```python
from build123d import *


with BuildPart() as f3:
    # F3: sweep along a path in F0
    with BuildLine(Plane.XZ) as f3_path:
        Line((-75.8256912231, 30), (74.0892291069, 30))
        ThreePointArc((74.0892291069, 30), (104.0892291069, 0), (74.0892291069, -30))
        Line((74.0892291069, -30), (-75.8256912231, -30))
        ThreePointArc((-75.8256912231, -30), (-105.8256912231, 0), (-75.8256912231, 30))
    # F2 (on plane+point) → F3 (sweep)
    with BuildSketch(Plane.YZ.offset(74.0892291069)):
        Polygon((1.443375673, 35), (2.8867513459, 32.5), (4.3301270189, 35), align=None)
        Polygon((-1.443375673, 35), (1.443375673, 35), (0, 37.5), align=None)
        Polygon((-4.3301270189, 35), (-2.8867513459, 32.5), (-1.443375673, 35), align=None)
        Polygon((-4.3301270189, 30), (-1.443375673, 30), (-2.8867513459, 32.5), align=None)
        Polygon((0, 27.5), (1.443375673, 30), (-1.443375673, 30), align=None)
        Polygon((1.443375673, 30), (4.3301270189, 30), (2.8867513459, 32.5), align=None)
        Polygon((-1.443375673, 30), (1.443375673, 30), (2.8867513459, 32.5), (1.443375673, 35), (-1.443375673, 35), (-2.8867513459, 32.5), align=None)
    sweep(path=f3_path.line)


solid = f3.part
```
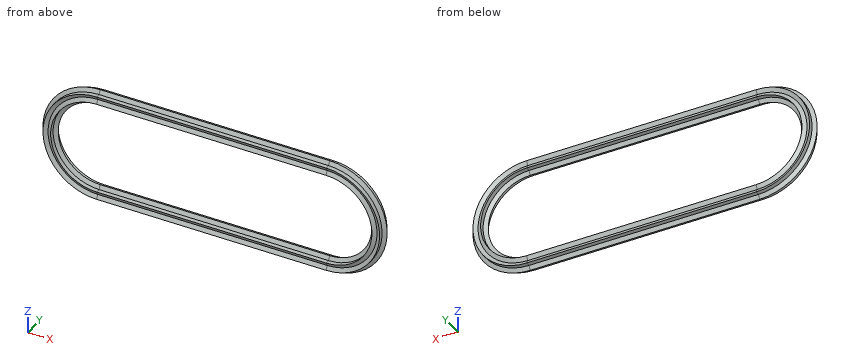
The listing builds one solid part. Answer for the finished solid, in the listing's coordinates (mm). Round coordinates to 2 decimals unless told otherwise and drop trailing zeros. Write each loop counter-clockwise with the first axis right and the second up, starting at its lowest first coordinate (ties: lowest second). Pieces come first, ordered by that corner, then holes. Notation, with made-up numbers: (22, 55) -> (57, 55) arc R19 ccw to (57, 75) -> close; hole circle Ø9 at (-28, 64.5). An arc over 180 degrees is marked (long way). Answer as a JSON object with one key per item and string values. Group by question number.
Q1. Each of these flat-tipped pins is pushed along its axis until it touches: pin 1 Ø2.5 at (x, y) = (-5.5, 3) entering from +Z; pin 2 Ø0.9 at (x, y) = (-25.5, 3) entering from -Z; pin 3 Ø2.5 at (x, y) = (20.5, -2.5) entering from +Z. Where does it stop, or does it pass through?
Q2. Section B-B (z = 0) is taken. Write down the section's boundary in (x, y), plus the area to 3 significant figures.
Q3. Straight lines are drawn through the part: line 1 along Z through (x, y) = (-28.5, -2.75); line 2 along Z through (x, y) = (-37.5, -3); line 3 along Z through (x, y) = (74, -3.25). For each, find the intervals that lie inside material, in ascending order.
Q4. Section A-A (x = -66) is taken. Write down the section's boundary in (y, z), plus the area to 3 significant figures.
Check values:
{
 "1": {"pin 1": "z = 35", "pin 2": "z = -35", "pin 3": "z = 35.33"},
 "2": {"outline": "(-113.33, 0) -> (-110.83, -1.44) -> (-110.83, -4.33) -> (-108.33, -2.89) -> (-105.83, -4.33) -> (-105.83, -1.44) -> (-103.33, 0) -> (-105.83, 1.44) -> (-105.83, 4.33) -> (-108.33, 2.89) -> (-110.83, 4.33) -> (-110.83, 1.44) -> close; (101.59, 0) -> (104.09, -1.44) -> (104.09, -4.33) -> (106.59, -2.89) -> (109.09, -4.33) -> (109.09, -1.44) -> (111.59, 0) -> (109.09, 1.44) -> (109.09, 4.33) -> (106.59, 2.89) -> (104.09, 4.33) -> (104.09, 1.44) -> close", "area": "86.6 mm^2"},
 "3": {"line 1": "-35 to -30, 30 to 35", "line 2": "-35 to -32.7, -32.3 to -30, 30 to 32.3, 32.7 to 35", "line 3": "-35 to -33.13, -31.87 to -30, 30 to 31.87, 33.13 to 35"},
 "4": {"outline": "(-4.33, -35) -> (-1.44, -35) -> (0, -37.5) -> (1.44, -35) -> (4.33, -35) -> (2.89, -32.5) -> (4.33, -30) -> (1.44, -30) -> (0, -27.5) -> (-1.44, -30) -> (-4.33, -30) -> (-2.89, -32.5) -> close; (-4.33, 30) -> (-1.44, 30) -> (0, 27.5) -> (1.44, 30) -> (4.33, 30) -> (2.89, 32.5) -> (4.33, 35) -> (1.44, 35) -> (0, 37.5) -> (-1.44, 35) -> (-4.33, 35) -> (-2.89, 32.5) -> close", "area": "86.6 mm^2"}
}
